Design review of the part shown in the three views and the two pictorial views. Dimensions are in mm from the part's minimum x, y and z. Give positions to 0.01 mm unless a question says otherwise; leave off trailing zeros. Order: outer loops, then holes, each group sorted by start corner. A loop starts at its lowest first (then second) coordinate and runs counter-clockwise, first axis right, second up. Notation, with made-up numbers: M 45.25,-8.5 L 84.25,-8.5 A31 ccw 84.25,19.5 Z; hole C 85,-15 d2. An arc over 180 degrees is marked long. Answer as a JSON object with one key per item and string values.
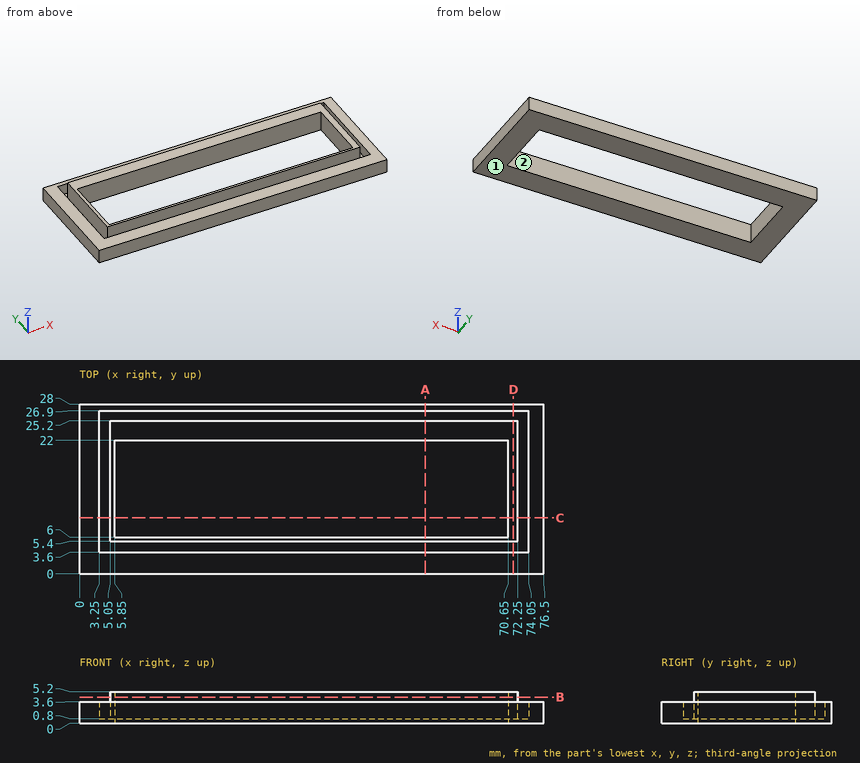
(1) Draft analysis for pull direction X (two halves, no side actions). For the marked faces 1 and 2, state which applies: +X half, -X half, draft (parallel to the pull), parting line (faces both ways), or undercut.
Checked values:
{"face 1": "draft", "face 2": "undercut"}
(2) Insertion check: pin 1 (2 mm diameter, centred on x = 68.5, y = 3.5, fed in from +Z). The pin has a flat end and moves straight along its axis. Give the tip position at first contact, or say it passes through.
Checked values:
{"pin 1": "stops at z = 3.6"}
(3) We need section A-A (x = 57). Write out the cut boundary in (y, z).
Checked values:
{"outline": "M 0,0 L 6,0 L 6,5.2 L 5.4,5.2 L 5.4,0.8 L 3.6,0.8 L 3.6,3.6 L 0,3.6 Z; M 22,0 L 28,0 L 28,3.6 L 26.9,3.6 L 26.9,0.8 L 25.2,0.8 L 25.2,5.2 L 22,5.2 Z"}
(4) We need section D-D (x = 71.5). Write out the cut boundary in (y, z).
Checked values:
{"outline": "M 0,0 L 28,0 L 28,3.6 L 26.9,3.6 L 26.9,0.8 L 25.2,0.8 L 25.2,5.2 L 5.4,5.2 L 5.4,0.8 L 3.6,0.8 L 3.6,3.6 L 0,3.6 Z"}
(5) To check wall thickness, follow L1, parallel to X at y = 9.25, z = 1.1; L2, parallel to Y at x = 71, z = 2.6; L3, parallel to Y at x = 26.5, z = 1.55. State the ranges of each line that lie inside material, in increasing order. Write a range as from..to.
Checked values:
{"L1": "x = 0..3.25, 5.05..5.85, 70.65..72.25, 74.05..76.5", "L2": "y = 0..3.6, 5.4..25.2, 26.9..28", "L3": "y = 0..3.6, 5.4..6, 22..25.2, 26.9..28"}
(6) We need section C-C (y = 9.25). Write out the cut boundary in (x, z).
Checked values:
{"outline": "M 0,0 L 5.85,0 L 5.85,5.2 L 5.05,5.2 L 5.05,0.8 L 3.25,0.8 L 3.25,3.6 L 0,3.6 Z; M 70.65,0 L 76.5,0 L 76.5,3.6 L 74.05,3.6 L 74.05,0.8 L 72.25,0.8 L 72.25,5.2 L 70.65,5.2 Z"}
(7) We need section B-B (z = 4.35). Write out the cut boundary in (x, y).
Checked values:
{"outline": "M 5.05,5.4 L 72.25,5.4 L 72.25,25.2 L 5.05,25.2 Z; hole M 5.85,6 L 70.65,6 L 70.65,22 L 5.85,22 Z"}
